Answer from the drawing. Dimensions are ordinates in mm from the lowest x, y and z of the part. Coordinates: 2 decimals unless noted, no trailing zeros. Write each loop counter-clockwise with the first axis right and the second up, starting at its lowest first coordinate (ties: lowest second). Pieces come first, ordered by that corner, then holes. Notation, with made-up numbers: (75.25, 35) - (106.25, 35) arc R34 cw to (106.25, 70) - close; hole circle Ø9 at (-11.5, 70). An arc over 180 degrees is marked (long way). Use a Markdown table: item, result.
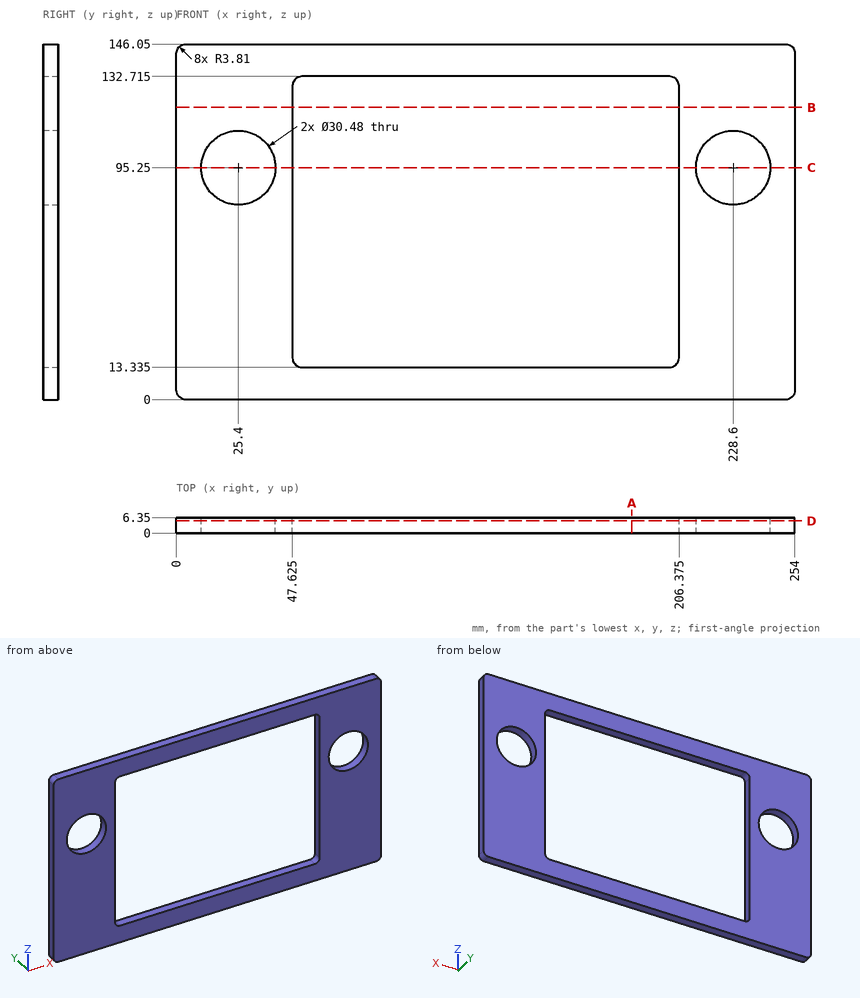
(1) This flat-tipped pin is pushed along its axis until it touches: P1, Ø1.5, axis at x = 205, z = 119.5, coming from the +Y side. Where does it stop, or does it pass through?
Report:
| item | result |
|---|---|
| P1 | passes through |
(2) A cutting plane is placed at A-A, the plane x = 187. Write down the section's boundary in (y, z) (3 decimals), and give its area (3 significant figures).
Report:
| item | result |
|---|---|
| outline | (0, 0) - (6.35, 0) - (6.35, 13.335) - (0, 13.335) - close; (0, 132.715) - (6.35, 132.715) - (6.35, 146.05) - (0, 146.05) - close |
| area | 169 mm² |
(3) A cutting plane is placed at C-C, the plane z = 95.25. Write down the section's boundary in (x, y) (3 decimals), and give its area (3 significant figures).
Report:
| item | result |
|---|---|
| outline | (0, 0) - (10.16, 0) - (10.16, 6.35) - (0, 6.35) - close; (40.64, 0) - (47.625, 0) - (47.625, 6.35) - (40.64, 6.35) - close; (206.375, 0) - (213.36, 0) - (213.36, 6.35) - (206.375, 6.35) - close; (243.84, 0) - (254, 0) - (254, 6.35) - (243.84, 6.35) - close |
| area | 218 mm² |
(4) Straight lines are drawn through the part: L1, parallel to X at y = 1.75, z = 95.25 (3 decimals); L2, parallel to X at y = 3.75, z = 54 (3 decimals); L3, parallel to Z at x = 106, y = 6 (3 decimals). For each, find the intervals that lie inside material, in ascending order.
Report:
| item | result |
|---|---|
| L1 | x = 0 to 10.16, 40.64 to 47.625, 206.375 to 213.36, 243.84 to 254 |
| L2 | x = 0 to 47.625, 206.375 to 254 |
| L3 | z = 0 to 13.335, 132.715 to 146.05 |
(5) A cutting plane is placed at B-B, the plane z = 120. Write down the section's boundary in (x, y) (3 decimals).
Report:
| item | result |
|---|---|
| outline | (0, 0) - (47.625, 0) - (47.625, 6.35) - (0, 6.35) - close; (206.375, 0) - (254, 0) - (254, 6.35) - (206.375, 6.35) - close |
(6) A cutting plane is placed at D-D, the plane y = 5. Write down the section's boundary in (x, z) (3 decimals).
Report:
| item | result |
|---|---|
| outline | (0, 3.81) arc R3.81 ccw to (3.81, 0) - (250.19, 0) arc R3.81 ccw to (254, 3.81) - (254, 142.24) arc R3.81 ccw to (250.19, 146.05) - (3.81, 146.05) arc R3.81 ccw to (0, 142.24) - close; hole circle Ø30.48 at (25.4, 95.25); hole (47.625, 17.145) arc R3.81 ccw to (51.435, 13.335) - (202.565, 13.335) arc R3.81 ccw to (206.375, 17.145) - (206.375, 128.905) arc R3.81 ccw to (202.565, 132.715) - (51.435, 132.715) arc R3.81 ccw to (47.625, 128.905) - close; hole circle Ø30.48 at (228.6, 95.25) |
